Can you work these out from the drawing? Everything is in mm from the part's minimum corner. Give positions to 0.01 mm unless a question says otherwise; leave off trailing zeros. Write each loop counter-clockwise with the first axis right and the second up, starting at its lowest first coordinate (ties: lowest second). Pieces come first, ordered by that corner, then holes. Notation, with made-up numbers: (73.5, 27) -> (106.5, 27) arc R22 cw to (106.5, 56) -> close; hole circle Ø10 at (19.5, -14). An arc over 180 degrees is marked (long way). Use one line per item in the form item = value.
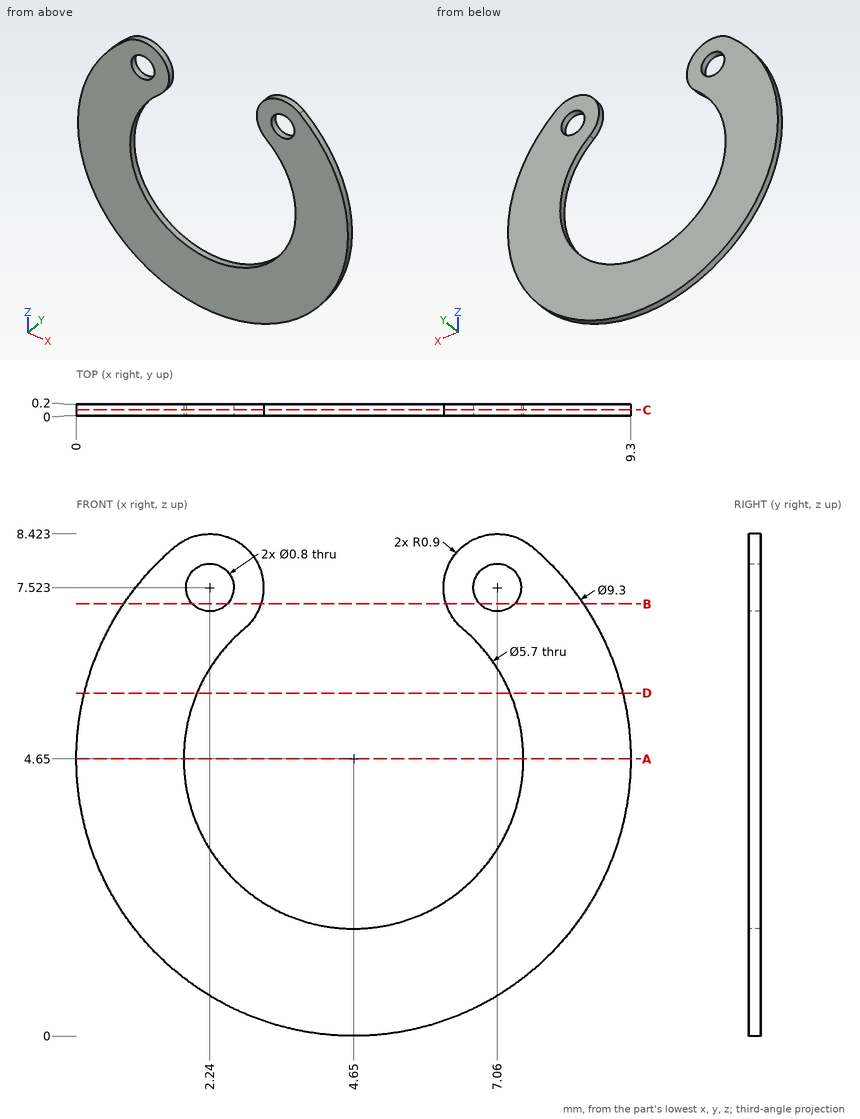
Q1. I want a section at B-B, the plane z = 7.25. Count the separate pieces of the cut face and the enclosed holes in it.
Result set:
separate_pieces = 4
enclosed_holes = 0
Q2. I want a section at D-D, the plane z = 5.75. Write out the boundary of the cut face in (x, y).
Result set:
outline = (0.13, 0) -> (2.02, 0) -> (2.02, 0.2) -> (0.13, 0.2) -> close; (7.28, 0) -> (9.17, 0) -> (9.17, 0.2) -> (7.28, 0.2) -> close
Q3. If I drill on line 1 along X through (y, z) = (0.05, 7.25) (1 decimal); line 2 along X through (y, z) = (0.15, 4.65); line 3 along Z through (x, y) = (7, 0.1) (1 decimal), over which ranges is the centre line in solid material (lowest first)? Write a range as from..to.
Result set:
line_1 = 0.8..1.9, 2.5..3.1, 6.2..6.8, 7.4..8.5
line_2 = 0..1.8, 7.5..9.3
line_3 = 0.6..3, 6.3..7.1, 7.9..8.4
Q4. I want a section at C-C, the plane y = 0.1. Write out the boundary of the cut face in (x, z).
Result set:
outline = (1.66, 8.21) arc R4.65 ccw (long way) to (7.64, 8.21) arc R0.9 ccw to (6.48, 6.83) arc R2.85 cw (long way) to (2.82, 6.83) arc R0.9 ccw to start; hole circle Ø0.8 at (2.24, 7.52); hole circle Ø0.8 at (7.06, 7.52)
Q5. I want a section at A-A, the plane z = 4.65. Write out the boundary of the cut face in (x, y).
Result set:
outline = (0, 0) -> (1.8, 0) -> (1.8, 0.2) -> (0, 0.2) -> close; (7.5, 0) -> (9.3, 0) -> (9.3, 0.2) -> (7.5, 0.2) -> close
